Read the model definition and answer for the solid it produces. Units are mm, in the model's axes. Face numbers are marked on the shaded views. A direction names the side the tool comes from. Give positions to 0.01 mm unless a question says otherwise; leave off trailing zeros. Order: outer loops, then holes, each group sorted by start corner. A loop starts at its lowest first (then second) coordinate and runs counter-clockwise, first axis right, second up. Notation, with made-up numbers: (44, -18) -> (70, -18) arc R22 ccw to (70, 10) -> close; hole circle Ø11 at (-20.5, 46). An arc over 180 degrees is marked (long way). Use one line per item in the form item = value.
Autodesk Inventor part; units mm, degrees
ref_plane "YZ Plane" through (0, 0, 0) normal (1, 0, 0) x (0, 1, 0)
ref_plane "XZ Plane" through (0, 0, 0) normal (0, 1, 0) x (-1, 0, 0)
ref_plane "XY Plane" through (0, 0, 0) normal (0, 0, 1) x (1, 0, 0)
sketch "Skizze61" plane through (0, 0, 0) normal (0, 0, 1) x (1, 0, 0)
  line L0 (30, -45) -> (-30, -45)
  line L1 (-30, -45) -> (-30, 45)
  line L2 (-30, 45) -> (30, 45)
  line L3 (30, 45) -> (30, -45)
  line L4 (30, -45) -> (-30, 45) construction
  line L5 (-30, -45) -> (30, 45) construction
  point P0 (0, 0)
  dimension "d159" = 60
  dimension "d160" = 90
extrude "Extrusion54" add sketch "Skizze61" along normal blind 65
shell "Wandung3" thickness 5 removed faces 1 at (-10, 15, 65)
sketch "Sketch69" plane through (-30, -45, 0) normal (-1, 0, 0) x (0, 0, 1)
  line L0 (0, 90) -> (65, 90)
  line L1 (0, 0) -> (65, 0)
  line L2 (0, 90) -> (10, 90)
  line L3 (10, 90) -> (10, 0)
  line L4 (10, 0) -> (0, 0)
  line L5 (0, 0) -> (0, 90)
  point P0 (0, 45)
  dimension "d192" = 10
extrude "Extrusion61" add sketch "Sketch69" along normal blind 59
sketch "Sketch71" plane through (0, 0, 0) normal (0, 0, -1) x (-1, 0, 0)
  line L0 (-8, -33.57) -> (-12, -33.57)
  line L1 (-12, -33.57) -> (-12, -26.57)
  line L2 (-12, -26.57) -> (-8, -26.57)
  line L3 (-8, -26.57) -> (-8, -33.57)
  line L4 (89, 45) -> (89, -45)
  line L5 (-30, -45) -> (89, -45)
  point P0 (0, 0)
  dimension "d199" = 4
  dimension "d200" = 7
  dimension "d201" = 97
  dimension "d202" = 11.43
extrude "Extrusion63" cut sketch "Sketch71" against normal blind 10
sketch "Sketch70" plane through (0, 0, 0) normal (0, 0, -1) x (-1, 0, 0)
  line L0 (30, 45) -> (89, 45)
  line L1 (30, -45) -> (89, -45)
  line L2 (89, 45) -> (69, 45)
  line L3 (69, 45) -> (69, -45)
  line L4 (69, -45) -> (89, -45)
  line L5 (89, -45) -> (89, 45)
  circle A0 centre (79, 0) radius 3
  point P0 (0, 0)
  dimension "d195" = 20
  dimension "d196" = 6
extrude "Extrusion62" cut sketch "Sketch70" against normal through all contours A0
sketch "Sketch72" plane through (0, 0, 0) normal (0, 0, -1) x (-1, 0, 0)
  circle A0 centre (-20, 0) radius 3
  line L0 (-30, -45) -> (-30, 45)
  point P0 (0, 0)
  dimension "d205" = 6
  dimension "d206" = 10
extrude "Extrusion64" cut sketch "Sketch72" against normal through all
sketch "Sketch73" plane through (0, 0, 0) normal (0, 0, -1) x (-1, 0, 0)
  point P0 (0, 0)
fillet "Rundung1" radius 15 2 edges at (-89, 45, 5) (-89, -45, 5)
fillet "Rundung2" radius 15 1 edges at (30, -45, 32.5)
sketch "Skizze78" plane through (-25, 40, 5) normal (0, 0, 1) x (1, 0, 0)
  line L0 (0, 0) -> (7, 0)
  line L1 (7, 0) -> (7, -7)
  line L2 (7, -7) -> (0, -7)
  line L3 (0, -7) -> (0, 0)
  line L4 (50, -80) -> (50, 0)
  line L5 (50, 0) -> (43, 0)
  line L6 (43, 0) -> (43, -7)
  line L7 (43, -7) -> (50, -7)
  line L8 (50, -7) -> (50, 0)
  line L9 (50, -80) -> (0, -80)
  line L10 (0, -80) -> (7, -80)
  line L11 (7, -80) -> (7, -73)
  line L12 (7, -73) -> (0, -73)
  line L13 (0, -73) -> (0, -80)
  line L14 (50, -80) -> (43, -80)
  line L15 (43, -80) -> (43, -73)
  line L16 (43, -73) -> (50, -73)
  line L17 (50, -73) -> (50, -80)
  point P0 (25, -40)
  dimension "d239" = 7
  dimension "d240" = 7
  dimension "d241" = 7
  dimension "d242" = 7
  dimension "d243" = 7
  dimension "d244" = 7
  dimension "d245" = 7
  dimension "d246" = 7
extrude "Extrusion68" add sketch "Skizze78" along normal up to surface (60 mm away)
sketch "Skizze79" plane through (0, 0, 65) normal (0, 0, 1) x (1, 0, 0)
  line L0 (30, 45) -> (-30, 45)
  line L1 (-30, -45) -> (15, -45)
  line L2 (-30, 45) -> (-28, 45)
  line L3 (-28, 45) -> (-28, -45)
  line L4 (-28, -45) -> (-30, -45)
  line L5 (-30, -45) -> (-30, 45)
  line L6 (30, -30) -> (30, 45)
  line L7 (-28, 45) -> (30, 45)
  line L8 (30, 45) -> (30, 43)
  line L9 (30, 43) -> (-28, 43)
  line L10 (-28, 43) -> (-28, 45)
  line L11 (30, 43) -> (28, 43)
  line L12 (28, 43) -> (28, -30)
  line L13 (28, -30) -> (30, -30)
  line L14 (30, -30) -> (30, 43)
  line L15 (-28, -45) -> (15, -45)
  line L16 (15, -45) -> (15, -43)
  line L17 (15, -43) -> (-28, -43)
  line L18 (-28, -43) -> (-28, -45)
  arc A0 (15, -45) -> (30, -30) centre (15, -30) ccw
  arc A1 (15, -45) -> (30, -30) centre (15, -30) ccw
  arc A2 (15, -43) -> (28, -30) centre (15, -30) ccw
  point P0 (0, 0)
  point P1 (-28, -43)
  point P2 (29, -30)
  dimension "d249" = 2
  dimension "d250" = 2
  dimension "d251" = 2
  dimension "d252" = 2
  dimension "d268" = 75
extrude "Extrusion69" add sketch "Skizze79" along normal blind 2 contours L6 L9 L3 L0 | L3 L1 L5 L0 | L6 L13 L12 L9 | A0 L16 A2 L13 | L17 L16 L1 L3
sketch "Skizze80" plane through (-18, -40, 5) normal (0, 0, 1) x (1, 0, 0)
  line L0 (0, 80) -> (36, 80)
  line L1 (0, 80) -> (6, 80)
  line L2 (6, 80) -> (6, 67)
  line L3 (6, 67) -> (0, 67)
  line L4 (0, 67) -> (0, 80)
  line L5 (-7, 7) -> (-7, 73)
  line L6 (0, 67) -> (-7, 67)
  line L7 (-7, 67) -> (-7, 73)
  line L8 (-7, 73) -> (0, 73)
  line L9 (0, 73) -> (0, 67)
  line L10 (36, 73) -> (36, 80)
  line L11 (36, 80) -> (30, 80)
  line L12 (30, 80) -> (30, 67)
  line L13 (30, 67) -> (36, 67)
  line L14 (36, 67) -> (36, 80)
  line L15 (43, 7) -> (43, 73)
  line L16 (36, 67) -> (43, 67)
  line L17 (43, 67) -> (43, 73)
  line L18 (43, 73) -> (36, 73)
  line L19 (36, 73) -> (36, 67)
  line L20 (-7, 7) -> (6, 7)
  line L21 (6, 7) -> (6, 13)
  line L22 (6, 13) -> (-7, 13)
  line L23 (-7, 13) -> (-7, 7)
  line L24 (36, 0) -> (0, 0)
  line L25 (6, 7) -> (0, 7)
  line L26 (0, 7) -> (0, 0)
  line L27 (0, 0) -> (6, 0)
  line L28 (6, 0) -> (6, 7)
  line L29 (43, 7) -> (30, 7)
  line L30 (30, 7) -> (30, 13)
  line L31 (30, 13) -> (43, 13)
  line L32 (43, 13) -> (43, 7)
  line L33 (36, 0) -> (30, 0)
  line L34 (30, 0) -> (30, 7)
  line L35 (30, 7) -> (36, 7)
  line L36 (36, 7) -> (36, 0)
  point P0 (18, 40)
  point P1 (43, 7)
  point P2 (43, 13)
  point P3 (30, 0)
  point P4 (-7, 13)
  point P5 (6, 0)
  point P6 (36, 73)
  point P7 (0, 73)
  point P8 (-7, 67)
  dimension "d255" = 6
  dimension "d256" = 13
  dimension "d257" = 6
  dimension "d258" = 13
  dimension "d259" = 7
  dimension "d260" = 6
  dimension "d261" = 13
  dimension "d262" = 6
  dimension "d263" = 6
  dimension "d264" = 13
  dimension "d265" = 6
  dimension "d274" = 13
extrude "Extrusion70" add sketch "Skizze80" along normal blind 10 contours L0 L2 L3 L4 | L4 L6 L5 L8 | L0 L10 L14 L13 L12 | L18 L15 L16 L14 | L22 L21 L20 L5 | L15 L29 L30 L31 | L20 L28 L24 L26 | L36 L24 L34 L29
sketch "Skizze81" plane through (0, 0, 65) normal (0, 0, 1) x (1, 0, 0)
  circle A0 centre (-21.7, -36.7) radius 2
  line L0 (-18, -33) -> (-18, -40)
  line L1 (-25, -33) -> (-18, -33)
  point P0 (0, 0)
  dimension "d269" = 3.7
  dimension "d270" = 3.7
  dimension "d271" = 4
extrude "Extrusion71" cut sketch "Skizze81" against normal blind 7
mirror "Spiegeln11" about plane through (0, 0, 0) normal (1, 0, 0) of "Extrusion71"
mirror "Spiegeln12" about plane through (0, 0, 0) normal (0, 1, 0) of "Extrusion71", "Spiegeln11"
sketch "Skizze82" plane through (-18, -40, 15) normal (0, 0, 1) x (1, 0, 0)
  circle A0 centre (33.7, 9.3) radius 2
  line L0 (30, 13) -> (30, 0)
  line L1 (43, 13) -> (30, 13)
  point P0 (18, 40)
  dimension "d275" = 4
  dimension "d276" = 3.7
  dimension "d277" = 3.7
extrude "Extrusion72" cut sketch "Skizze82" against normal blind 7
mirror "Spiegeln13" about plane through (0, 0, 0) normal (0, 1, 0) of "Extrusion72"
mirror "Spiegeln14" about plane through (0, 0, 0) normal (1, 0, 0) of "Extrusion72", "Spiegeln13"
properties part number "Gehäuse"
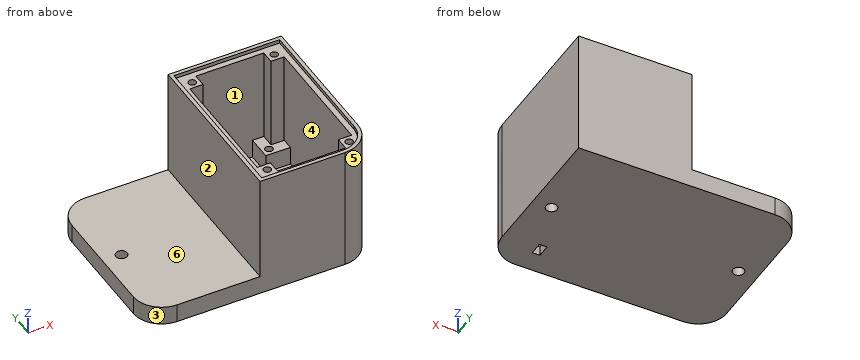
Item 1: Which of the six approach directions +Z, -Z, +X, -X, +Y, -Y give full straight-line access (tool end or side, diameter ignored) to the marked faces 5 and 6?
Checks:
face_5 = +Z, -Z, +X, -Y
face_6 = +Z, -X, +Y, -Y
Item 2: The part is cut by section B-B on x = -10. Give the vertices of the cut face in (y, z).
Checks:
outline = (-45, 0) -> (45, 0) -> (45, 67) -> (43, 67) -> (43, 65) -> (40, 65) -> (40, 5) -> (-40, 5) -> (-40, 65) -> (-43, 65) -> (-43, 67) -> (-45, 67) -> close
Item 3: Given pin 1 Ø2 at (x, y) = (-58.5, -28.5) entering from +Z; pin 2 Ø5 at (x, y) = (20, 0) entering from -Z; pin 3 Ø7.5 at (x, z) = (23, 37.5) entering from -Y; pin 4 Ø7.5 at (y, z) = (-37.5, 36) entering from +X, each flat-ended and moving along its own axis, determine where each tip first touches the part or whether it passes through.
Checks:
pin_1 = 10
pin_2 = through
pin_3 = -44.39
pin_4 = 29.52
Item 4: The part is cut by section A-A on z = 36.5. Give the vertices of the cut face in (x, y), and give its area (3 significant figures).
Checks:
outline = (-30, -45) -> (15, -45) arc R15 ccw to (30, -30) -> (30, 45) -> (-30, 45) -> close; hole (-25, -33) -> (-18, -33) -> (-18, -40) -> (18, -40) -> (18, -33) -> (25, -33) -> (25, 33) -> (18, 33) -> (18, 40) -> (-18, 40) -> (-18, 33) -> (-25, 33) -> close
area = 1,550 mm²
Item 5: The part is cut by section C-C on z = 61. Give the vertices of the cut face in (x, y).
Checks:
outline = (-30, -45) -> (15, -45) arc R15 ccw to (30, -30) -> (30, 45) -> (-30, 45) -> close; hole (-25, -33) -> (-18, -33) -> (-18, -40) -> (18, -40) -> (18, -33) -> (25, -33) -> (25, 33) -> (18, 33) -> (18, 40) -> (-18, 40) -> (-18, 33) -> (-25, 33) -> close; hole circle Ø4 at (-21.7, -36.7); hole circle Ø4 at (-21.7, 36.7); hole circle Ø4 at (21.7, -36.7); hole circle Ø4 at (21.7, 36.7)
Item 6: The part is cut by section D-D on y = -16.5. Give the vertices of the cut face in (x, z), and give its area (3 significant figures).
Checks:
outline = (-89, 0) -> (30, 0) -> (30, 67) -> (28, 67) -> (28, 65) -> (25, 65) -> (25, 5) -> (-25, 5) -> (-25, 65) -> (-28, 65) -> (-28, 67) -> (-30, 67) -> (-30, 10) -> (-89, 10) -> close
area = 1,500 mm²
Item 7: Determine the mould class of the marked faces 1, 2, 3 and 4 for opening direction Y: +Y half, -Y half, draft (parallel to the pull), parting line (faces both ways), or undercut.
Checks:
face_1 = undercut
face_2 = draft
face_3 = -Y half
face_4 = undercut
Item 8: Straight lines are drawn through the part: L1, parallel to X at y = -17.5, z = 43; L2, parallel to X at y = 36.7, z = 62.75; L3, parallel to X at y = -30, z = 12. For each, find the intervals that lie inside material, in ascending order. Write a range as from..to.
Checks:
L1 = -30..-25, 25..30
L2 = -30..-23.7, -19.7..-18, 18..19.7, 23.7..30
L3 = -30..-17.57, -13.83..-12, 12..13.83, 17.57..30
